from build123d import *

# Parameters (mm, degrees)
SKIZZE1_W                       = 42.3
SKIZZE1_H                       = 42.3
AUFSATZ_LINEAR_AUSTRAGEN1_DEPTH = 34
SKIZZE2_R                       = 18
AUFSATZ_LINEAR_AUSTRAGEN2_DEPTH = 27.3
SKIZZE3_R                       = 11
AUFSATZ_LINEAR_AUSTRAGEN3_DEPTH = 2
SKIZZE4_R                       = 7.5
AUFSATZ_LINEAR_AUSTRAGEN4_DEPTH = 1
SKIZZE5_R                       = 3
AUFSATZ_LINEAR_AUSTRAGEN5_DEPTH = 15
SCHNITT_LINEAR_START            = -12
SCHNITT_LINEAR_AUSTRAGEN1_DEPTH = 12
M3_GEWINDEBOHRUNG1_D            = 2.5
M3_GEWINDEBOHRUNG1_DEPTH        = 8.5
M3_GEWINDEBOHRUNG1_TIP          = 0.751075774
SKIZZE9_R                       = 5.5
AUFSATZ_LINEAR_AUSTRAGEN6_DEPTH = 5


with BuildPart() as part:
    # Skizze1 → Aufsatz-Linear austragen1 (new body)
    with BuildSketch(Plane.XY):
        with Locations((21.15, 21.15)):
            Rectangle(SKIZZE1_W, SKIZZE1_H)
    extrude(amount=AUFSATZ_LINEAR_AUSTRAGEN1_DEPTH)

    # Skizze2 → Aufsatz-Linear austragen2 (add)
    with BuildSketch(Plane.XY.offset(34)):
        with Locations(Location((21.15, 21.15, 0), (0, 0, 180))):
            Circle(SKIZZE2_R)
    extrude(amount=AUFSATZ_LINEAR_AUSTRAGEN2_DEPTH)

    # Skizze3 → Aufsatz-Linear austragen3 (add)
    with BuildSketch(Plane.XY.offset(61.3)):
        with Locations((21.15, 21.15)):
            Circle(SKIZZE3_R)
    extrude(amount=AUFSATZ_LINEAR_AUSTRAGEN3_DEPTH)

    # Skizze4 → Aufsatz-Linear austragen4 (add)
    with BuildSketch(Plane.XY.offset(63.3)):
        with Locations((21.15, 21.15)):
            Circle(SKIZZE4_R)
    extrude(amount=AUFSATZ_LINEAR_AUSTRAGEN4_DEPTH)

    # Skizze5 → Aufsatz-Linear austragen5 (add)
    with BuildSketch(Plane.XY.offset(64.3)):
        with Locations((21.15, 21.15)):
            Circle(SKIZZE5_R)
    extrude(amount=AUFSATZ_LINEAR_AUSTRAGEN5_DEPTH)

    # Skizze6 → Schnitt-Linear austragen1 (cut)
    with BuildSketch(Plane.XY.offset(79.3).offset(SCHNITT_LINEAR_START)):
        with BuildLine():
            Line((23.386067977, 23.15), (18.913932023, 23.15))
            ThreePointArc((18.913932023, 23.15), (21.15, 24.15), (23.386067977, 23.15))
        make_face()
    extrude(amount=SCHNITT_LINEAR_AUSTRAGEN1_DEPTH, mode=Mode.SUBTRACT)

    # M3 Gewindebohrung1
    with Locations(Plane.XY.offset(61.3)):
        with Locations((11.250505063, 11.250505063), (31.049494937, 11.250505063), (31.049494937, 31.049494937), (11.250505063, 31.049494937)):
            Hole(M3_GEWINDEBOHRUNG1_D / 2, depth=M3_GEWINDEBOHRUNG1_DEPTH)
            with Locations((0, 0, -(M3_GEWINDEBOHRUNG1_DEPTH + M3_GEWINDEBOHRUNG1_TIP / 2))):  # 118° drill point
                Cone(0, M3_GEWINDEBOHRUNG1_D / 2, M3_GEWINDEBOHRUNG1_TIP, mode=Mode.SUBTRACT)

    # Skizze9 → Aufsatz-Linear austragen6 (add)
    with BuildSketch(Plane(origin=(0, 0, 0), x_dir=(-1, 0, 0), z_dir=(0, -1, 0))):
        with Locations(Location((-21.15, -10, 0), (0, 0, 270))):
            Circle(SKIZZE9_R)
    extrude(amount=AUFSATZ_LINEAR_AUSTRAGEN6_DEPTH)


solid = part.part
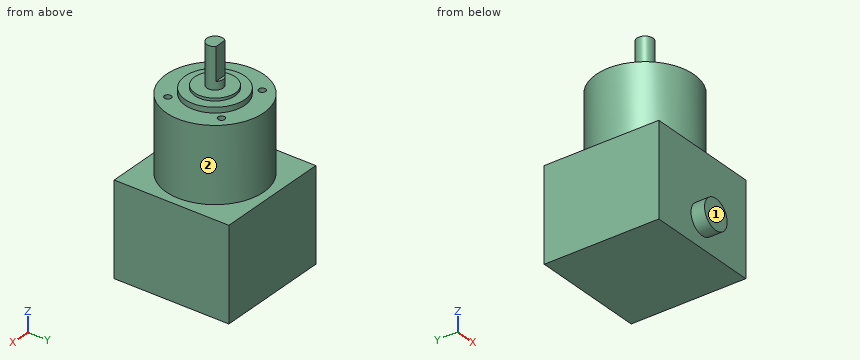
Model file for the job. Use its own axes, mm. Face numbers are marked on the shaded views. A direction names the side the tool comes from. Give positions to 0.01 mm unless a question says otherwise; leave off trailing zeros. Loops run counter-clockwise (first coordinate to the right, second up) from the corner with the lowest first, then second, coordinate; pieces in that order, holes last.
1) Wall check: line 1 (Y direction, x = 35.5, z = 7); line 2 (Z direction, x = 30, y = 18.5); line 3 (Z direction, x = 8.5, y = 16). Give the ranges that are in metal, low to high.
2) Saw through at A-A (y = 21.15). Write the cut outline in (x, z), plus the area to 3 significant figures.
3) Flat gauge pins, fed straight in: pin 1 Ø1.5 at (x, z) = (21.5, 41) entering from +Y; pin 2 Ø6 at (x, y) = (27, 30) entering from +Z; pin 3 Ø4 at (x, z) = (9.5, 35) entering from +Y; pin 4 Ø1.5 at (y, z) = (25, 51.5) entering from -X. Where does each tip first touch, or does it go through?
4) Saw through at D-D (x = 37). Write the cut outline in (y, z), plus the area to 3 significant figures.
5) Tool access for the marked faces 1 and 2: list every direction of +Z, -Z, +X, -X, +Y, -Y with a clear straight run to the whole face (end or side of a thin tool).
6) Saw through at B-B (z = 10). Write the cut outline in (x, y), plus the area to 3 significant figures.
7) Saw through at C-C (x = 21.15). Write the cut outline in (y, z), plus the area to 3 significant figures.
Answer block:
1. line 1: y = 0 to 42.3
1. line 2: z = 0 to 63.3
1. line 3: z = 0 to 61.3
2. outline: (0, 0) - (42.3, 0) - (42.3, 34) - (39.15, 34) - (39.15, 61.3) - (32.15, 61.3) - (32.15, 63.3) - (28.65, 63.3) - (28.65, 64.3) - (24.15, 64.3) - (24.15, 79.3) - (18.15, 79.3) - (18.15, 64.3) - (13.65, 64.3) - (13.65, 63.3) - (10.15, 63.3) - (10.15, 61.3) - (3.15, 61.3) - (3.15, 34) - (0, 34) - close
2. area: 2,570 mm2
3. pin 1: stops at y = 39.15
3. pin 2: stops at z = 63.3
3. pin 3: stops at y = 42.3
3. pin 4: stops at x = 3.42
4. outline: (0, 0) - (42.3, 0) - (42.3, 34) - (29.68, 34) - (29.68, 61.3) - (12.62, 61.3) - (12.62, 34) - (0, 34) - close
4. area: 1,900 mm2
5. face 1: +Z, -Z, +X, -X, -Y
5. face 2: +Z
6. outline: (0, 0) - (15.65, 0) - (15.65, -5) - (26.65, -5) - (26.65, 0) - (42.3, 0) - (42.3, 42.3) - (0, 42.3) - close
6. area: 1,840 mm2
7. outline: (-5, 4.5) - (0, 4.5) - (0, 0) - (42.3, 0) - (42.3, 34) - (39.15, 34) - (39.15, 61.3) - (32.15, 61.3) - (32.15, 63.3) - (28.65, 63.3) - (28.65, 64.3) - (24.15, 64.3) - (24.15, 67.3) - (23.15, 67.3) - (23.15, 79.3) - (18.15, 79.3) - (18.15, 64.3) - (13.65, 64.3) - (13.65, 63.3) - (10.15, 63.3) - (10.15, 61.3) - (3.15, 61.3) - (3.15, 34) - (0, 34) - (0, 15.5) - (-5, 15.5) - close
7. area: 2,610 mm2
